Build history of the part. All positions in model axes, mm. A direction names the side the tool comes from. Coordinates: 2 decimals unless noted, no trailing zeros. Write each loop counter-clockwise with the first axis right and the second up, starting at its lowest first coordinate (ties: lowest second). Pieces come first, ordered by that corner, then holes.
```python
from build123d import *

# Parameters (mm, degrees)
BASE_FLANGE1_DEPTH = 4
FILLET1_R          = 2
FILLET2_R          = 5
FILLET3_R          = 10
SKETCH6_R          = 1.6
CUT_EXTRUDE1_DEPTH = 10


# Sheet-metal steps are written as plain solids
with BuildPart() as part:
    # Sketch1 → Base-Flange1 (new body)
    with BuildSketch(Plane(origin=(0, 0, 0), x_dir=(1, 0, 0), z_dir=(0, 1, 0))):
        with BuildLine():
            Line((0, 0), (-5, 0))
            Line((-5, 0), (-5, 14.567226763))
            ThreePointArc((-5, 14.567226763), (-4.914448614, 15.872488686), (-4.659258263, 17.155417214))
            Line((-4.659258263, 17.155417214), (-2.411809549, 25.543010002))
            ThreePointArc((-2.411809549, 25.543010002), (-12.545541462, 29.253521737), (-8.119779436, 19.41111094))
            Line((-8.119779436, 19.41111094), (-8, 14.412545857))
            ThreePointArc((-8, 14.412545857), (-15.893198966, 32.982001696), (2.588190451, 24.884747514))
            Line((2.588190451, 24.884747514), (0.340741737, 16.497154727))
            ThreePointArc((0.340741737, 16.497154727), (0.085551386, 15.214226198), (0, 13.908964276))
            Line((0, 13.908964276), (0, 0))
        make_face()
    extrude(amount=-BASE_FLANGE1_DEPTH)

    # Fillet1
    fillet1_edges = [part.edges().sort_by_distance(p)[0] for p in [
        (-8.119779436, -2, -19.41111094),
        (-8, -2, -14.412545857),
    ]]
    fillet(fillet1_edges, radius=FILLET1_R)

    # Fillet2
    fillet2_edges = [part.edges().sort_by_distance(p)[0] for p in [
        (-2.411809549, -2, -25.543010002),
    ]]
    fillet(fillet2_edges, radius=FILLET2_R)

    # Fillet3
    fillet3_edges = [part.edges().sort_by_distance(p)[0] for p in [
        (2.588190451, -2, -24.884747514),
    ]]
    fillet(fillet3_edges, radius=FILLET3_R)

    # Sketch6 → Cut-Extrude1 (cut)
    with BuildSketch(Plane(origin=(0, 0, 0), x_dir=(1, 0, 0), z_dir=(0, 1, 0))):
        with Locations(Location((-2.5, 2.5, 0), (0, 0, 270))):
            Circle(SKETCH6_R)
    extrude(amount=-CUT_EXTRUDE1_DEPTH, mode=Mode.SUBTRACT)


solid = part.part
```
1. Saw through at A-A on z = -2.5. List the corners of the cut face in (x, y), plus the area to 3 significant figures.
Computed values:
outline: (-5, -4) - (-4.1, -4) - (-4.1, 0) - (-5, 0) - close; (-0.9, -4) - (0, -4) - (0, 0) - (-0.9, 0) - close
area: 7.20 mm2
2. Saw through at B-B on x = -2. List the corners of the cut face in (y, z).
Computed values:
outline: (-4, -34.13) - (0, -34.13) - (0, -4.02) - (-4, -4.02) - close; (-4, -0.98) - (0, -0.98) - (0, 0) - (-4, 0) - close
3. Saw through at D-D on z = -7.5. List the corners of the cut face in (x, y).
Computed values:
outline: (-5, -4) - (0, -4) - (0, 0) - (-5, 0) - close
4. Probe line 1 along X through (y, z) = (-2.8, -2.5); line 2 along X through (y, z) = (-2.6, -16); line 3 along X through (y, z) = (-3.2, -4.5). List the from-to ranges inside material, lowest first.
Computed values:
line 1: x = -5 to -4.1, -0.9 to 0
line 2: x = -13.92 to -8.14, -4.9 to 0.22
line 3: x = -5 to 0
5. Mould opens along X. For faces 1 (the face through (2.334, -2.028, -27.309)), 2 (the face through (-3, -4, -21)), 3 (the face through (-3.7, -1.97, -20.74)) say: +X half, -X half, draft (parallel to the pull), parting line (faces both ways), or undercut.
Computed values:
face 1: +X half
face 2: draft
face 3: undercut
6. Saw through at C-C on y = -0.95. List the corners of the cut face in (x, z).
Computed values:
outline: (-10.46, -14.63) arc R10.85 ccw (long way) to (0.89, -31.11) arc R10 ccw to (2.12, -23.14) - (0.34, -16.5) arc R10 cw to (0, -13.91) - (0, 0) - (-5, 0) - (-5, -14.57) arc R10 ccw to (-4.66, -17.16) - (-2.71, -24.43) arc R5 cw to (-3.33, -28.42) arc R5.85 cw (long way) to (-9.61, -19.57) arc R2 ccw to (-8.08, -17.67) - (-8.05, -16.64) arc R2 ccw to start; hole circle Ø3.2 at (-2.5, -2.5)
7. 3-axis set-ups, long thin cutter, end or side, ignore diameter. For faces 4 (the face through (0, -2, -7)), 5 (the face through (-2, -2, 0)), 6 (the face through (-3, 0, -21)), 7 (the face through (-8.535, -2.028, -18.895)), 8 (the face through (-5, -2, -7)): which of +Z, -Z, +X, -X, +Y, -Y reach the whole face in a straight line?
Computed values:
face 4: +Z, +X, +Y, -Y
face 5: +Z, +X, -X, +Y, -Y
face 6: +Z, -Z, +X, -X, +Y
face 7: +Y, -Y
face 8: +Z, -X, +Y, -Y
